from build123d import *

# Parameters (mm, degrees)
CROQUIS1_W              = 50
CROQUIS1_H              = 110
SALIENTE_EXTRUIR1_DEPTH = 4.5
REDONDEO1_R             = 2
CROQUIS2_R              = 3.5
CROQUIS2_R_2            = 2.6
SALIENTE_EXTRUIR2_DEPTH = 5
CROQUIS3_W              = 35
CROQUIS3_H              = 90
SALIENTE_EXTRUIR3_DEPTH = 23
CROQUIS5_W              = 30
CROQUIS5_H              = 21
CORTAR_EXTRUIR2_DEPTH   = 106.61249926
CORTAR_EXTRUIR4_DEPTH   = 10
CORTAR_EXTRUIR5_DEPTH   = 10


with BuildPart() as part:
    # Croquis1 → Saliente-Extruir1 (new body)
    with BuildSketch(Plane.XY):
        Rectangle(CROQUIS1_W, CROQUIS1_H)
    extrude(amount=SALIENTE_EXTRUIR1_DEPTH)

    # Redondeo1
    redondeo1_edges = [part.edges().sort_by_distance(p)[0] for p in [
        (-25, 0, 4.5),
        (0, -55, 4.5),
        (25, 0, 4.5),
        (0, -55, 0),
        (-25, 0, 0),
        (0, 55, 0),
        (25, 0, 0),
        (0, 55, 4.5),
    ]]
    fillet(redondeo1_edges, radius=REDONDEO1_R)

    # Croquis2 → Saliente-Extruir2 (add)
    # profile 1 of 16: a face of its own
    with BuildSketch(Plane.XY.offset(4.5)):
        with Locations(Location((-15, 50, 0), (0, 0, 121.002719134))):
            Circle(CROQUIS2_R)
        with Locations((-15, 50)):
            Circle(CROQUIS2_R_2, mode=Mode.SUBTRACT)
    # profile 2 of 16: a face of its own
    with BuildSketch(Plane.XY.offset(4.5)):
        with Locations((-15, 40)):
            Circle(CROQUIS2_R)
        with Locations((-15, 40)):
            Circle(CROQUIS2_R_2, mode=Mode.SUBTRACT)
    # profile 3 of 16: a face of its own
    with BuildSketch(Plane.XY.offset(4.5)):
        with Locations((-9, 45)):
            Circle(CROQUIS2_R)
        with Locations((-9, 45)):
            Circle(CROQUIS2_R_2, mode=Mode.SUBTRACT)
    # profile 4 of 16: a face of its own
    with BuildSketch(Plane.XY.offset(4.5)):
        with Locations(Location((-21, 45, 0), (0, 0, 235.150095421))):
            Circle(CROQUIS2_R)
        with Locations(Location((-21, 45, 0), (0, 0, 219.715137232))):
            Circle(CROQUIS2_R_2, mode=Mode.SUBTRACT)
    # profile 5 of 16: a face of its own
    with BuildSketch(Plane.XY.offset(4.5)):
        with Locations(Location((21, 45, 0), (0, 0, 180))):
            Circle(CROQUIS2_R)
        with Locations(Location((21, 45, 0), (0, 0, 180))):
            Circle(CROQUIS2_R_2, mode=Mode.SUBTRACT)
    # profile 6 of 16: a face of its own
    with BuildSketch(Plane.XY.offset(4.5)):
        with Locations(Location((15, 40, 0), (0, 0, 180))):
            Circle(CROQUIS2_R)
        with Locations(Location((15, 40, 0), (0, 0, 180))):
            Circle(CROQUIS2_R_2, mode=Mode.SUBTRACT)
    # profile 7 of 16: a face of its own
    with BuildSketch(Plane.XY.offset(4.5)):
        with Locations(Location((9, 45, 0), (0, 0, 180))):
            Circle(CROQUIS2_R)
        with Locations(Location((9, 45, 0), (0, 0, 180))):
            Circle(CROQUIS2_R_2, mode=Mode.SUBTRACT)
    # profile 8 of 16: a face of its own
    with BuildSketch(Plane.XY.offset(4.5)):
        with Locations(Location((15, 50, 0), (0, 0, 180))):
            Circle(CROQUIS2_R)
        with Locations(Location((15, 50, 0), (0, 0, 180))):
            Circle(CROQUIS2_R_2, mode=Mode.SUBTRACT)
    # profile 9 of 16: a face of its own
    with BuildSketch(Plane.XY.offset(4.5)):
        with Locations((15, -40)):
            Circle(CROQUIS2_R)
        with Locations((15, -40)):
            Circle(CROQUIS2_R_2, mode=Mode.SUBTRACT)
    # profile 10 of 16: a face of its own
    with BuildSketch(Plane.XY.offset(4.5)):
        with Locations(Location((21, -45, 0), (0, 0, 55.150095421))):
            Circle(CROQUIS2_R)
        with Locations(Location((21, -45, 0), (0, 0, 39.715137232))):
            Circle(CROQUIS2_R_2, mode=Mode.SUBTRACT)
    # profile 11 of 16: a face of its own
    with BuildSketch(Plane.XY.offset(4.5)):
        with Locations((9, -45)):
            Circle(CROQUIS2_R)
        with Locations((9, -45)):
            Circle(CROQUIS2_R_2, mode=Mode.SUBTRACT)
    # profile 12 of 16: a face of its own
    with BuildSketch(Plane.XY.offset(4.5)):
        with Locations(Location((15, -50, 0), (0, 0, 238.997280866))):
            Circle(CROQUIS2_R)
        with Locations((15, -50)):
            Circle(CROQUIS2_R_2, mode=Mode.SUBTRACT)
    # profile 13 of 16: a face of its own
    with BuildSketch(Plane.XY.offset(4.5)):
        with Locations(Location((-15, -40, 0), (0, 0, 180))):
            Circle(CROQUIS2_R)
        with Locations(Location((-15, -40, 0), (0, 0, 180))):
            Circle(CROQUIS2_R_2, mode=Mode.SUBTRACT)
    # profile 14 of 16: a face of its own
    with BuildSketch(Plane.XY.offset(4.5)):
        with Locations(Location((-9, -45, 0), (0, 0, 180))):
            Circle(CROQUIS2_R)
        with Locations(Location((-9, -45, 0), (0, 0, 180))):
            Circle(CROQUIS2_R_2, mode=Mode.SUBTRACT)
    # profile 15 of 16: a face of its own
    with BuildSketch(Plane.XY.offset(4.5)):
        with Locations(Location((-21, -45, 0), (0, 0, 180))):
            Circle(CROQUIS2_R)
        with Locations(Location((-21, -45, 0), (0, 0, 180))):
            Circle(CROQUIS2_R_2, mode=Mode.SUBTRACT)
    # profile 16 of 16: a face of its own
    with BuildSketch(Plane.XY.offset(4.5)):
        with Locations(Location((-15, -50, 0), (0, 0, 180))):
            Circle(CROQUIS2_R)
        with Locations(Location((-15, -50, 0), (0, 0, 180))):
            Circle(CROQUIS2_R_2, mode=Mode.SUBTRACT)
    extrude(amount=SALIENTE_EXTRUIR2_DEPTH)

    # Croquis3 → Saliente-Extruir3 (add)
    with BuildSketch(Plane(origin=(0, 0, 0), x_dir=(-1, 0, 0), z_dir=(0, 0, -1))):
        Rectangle(CROQUIS3_W, CROQUIS3_H)
    extrude(amount=SALIENTE_EXTRUIR3_DEPTH)

    # Croquis5 → Cortar-Extruir2 (cut, through all)
    with BuildSketch(Plane(origin=(0, 45, 0), x_dir=(1, 0, 0), z_dir=(0, 1, 0))):
        with Locations((0, 11.5)):
            Rectangle(CROQUIS5_W, CROQUIS5_H)
    extrude(amount=-CORTAR_EXTRUIR2_DEPTH, mode=Mode.SUBTRACT)

    # Croquis7 → Cortar-Extruir4 (cut)
    with BuildSketch(Plane.ZY.offset(17.5)):
        with BuildLine():
            add(Edge.make_bspline(
                [(-21.408360481, -7.762503909), (-17.763506305, -12.708708723), (-10.693467631, -23.108472428), (-3.641142742, -7.047797831)],
                knots=[0, 0, 0, 0, 1, 1, 1, 1], degree=3))
            add(Edge.make_bspline(
                [(-21.408360481, -7.762503909), (-21.767705448, -28.605682654), (-0.342880562, -25.676501046), (-3.641142742, -7.047797831)],
                knots=[0, 0, 0, 0, 1, 1, 1, 1], degree=3))
        make_face()
        Polygon((-5.763831244, 18.862685602), (-19.203160033, 12.99310964), (-7.830916468, 3.170101587), align=None)
        Polygon((-14.380375291, 20.063034513), (-16.287856832, 5.033414493), (-3.449369764, 10.442542671), align=None)
        Polygon((-14.380375291, 20.063034513), (-15.047295785, 14.808167615), (-10.611102479, 16.745658244), align=None)
        Polygon((-15.047295785, 14.808167615), (-19.203160033, 12.99310964), (-15.665473408, 9.937360437), align=None)
        Polygon((-12.053495915, 6.817440977), (-15.665473408, 9.937360437), (-16.287856832, 5.033414493), align=None)
        Polygon((-7.074130605, 8.915353688), (-12.053495915, 6.817440977), (-7.830916468, 3.170101587), align=None)
        Polygon((-5.763831244, 18.862685602), (-10.611102479, 16.745658244), (-6.517294779, 13.142655438), align=None)
        Polygon((-6.517294779, 13.142655438), (-7.074130605, 8.915353688), (-3.449369764, 10.442542671), align=None)
    extrude(amount=-CORTAR_EXTRUIR4_DEPTH, mode=Mode.SUBTRACT)

    # Croquis8 → Cortar-Extruir5 (cut)
    with BuildSketch(Plane(origin=(17.5, 0, 0), x_dir=(0, 0, -1), z_dir=(1, 0, 0))):
        with BuildLine():
            add(Edge.make_bspline(
                [(2.569348743, 40.716245485), (9.080503754, 18.53762373), (10.580801765, -9.48585487), (2.377628668, -42.298547258)],
                knots=[0, 0, 0, 0, 1, 1, 1, 1], degree=3))
            add(Edge.make_bspline(
                [(2.377628668, -42.298547258), (5.133604453, -15.937039747), (3.893375388, 16.552759214), (2.569348743, 40.716245485)],
                knots=[0, 0, 0, 0, 1, 1, 1, 1], degree=3))
        make_face()
        with BuildLine():
            add(Edge.make_bspline(
                [(20.430651257, 40.716245485), (13.919496246, 18.53762373), (12.419198235, -9.48585487), (20.622371332, -42.298547258)],
                knots=[0, 0, 0, 0, 1, 1, 1, 1], degree=3))
            add(Edge.make_bspline(
                [(20.622371332, -42.298547258), (17.866395547, -15.937039747), (19.106624612, 16.552759214), (20.430651257, 40.716245485)],
                knots=[0, 0, 0, 0, 1, 1, 1, 1], degree=3))
        make_face()
    extrude(amount=-CORTAR_EXTRUIR5_DEPTH, mode=Mode.SUBTRACT)


solid = part.part
The listing builds one solid part. Answer for the finished solid, in the listing's coordinates (mm). A direction names the side the tool comes from. Coordinates: 2 decimals unless noted, no trailing zeros. Write each loop counter-clockwise with the first axis right and the second up, starting at its lowest first coordinate (ties: lowest second). Pieces come first, ordered by that corner, then holes. Notation, with made-up numbers: M 19.5,75 L 50.5,75 A19 cw 50.5,79 Z; hole C -38,60 d7. An arc over 180 degrees is marked long. Write each question's results on one line, items separated by ' | '.
Item 1: Consider probe 1 along Z at (x, y) = (5.5, 40); probe 2 along Z at (x, y) = (6, 43.5); probe 3 along X at (y, z) = (-32, -8). Determine where each line is inside the solid, lowest interval first. Write a range as [from, to].
Answer below:
probe 1: [-23, -22], [-1, 4.5] | probe 2: [-23, -22], [-1, 9.5] | probe 3: [-17.5, -15], [15, 17.5]
Item 2: Which of the six approach directions +Z, -Z, +X, -X, +Y, -Y give full straight-line access (tool end or side, diameter ignored) to faces 3 (the face through (-16.27, 17.47, -14.71)), 4 (the face through (15, -37, 9.5)), 5 (the face through (-15, 1, -11)), 6 (the face through (21.46, 41.53, 6.96))?
Answer below:
face 3: -X | face 4: +Z, +X, -X, +Y, -Y | face 5: +Y, -Y | face 6: +Z
Item 3: For a pull along Y with two mould halves and no side action, classify faces 1 (the face through (22.19, -47.31, 6.96)), 2 (the face through (24.43, 0.77, 0.6)) as released by +Y, released by -Y, zero draft, split by the parting line, or undercut.
Answer below:
face 1: undercut | face 2: zero draft
Item 4: The part is cut by section D-D on x = -21. Determine the outline of the cut face in (y, z), and give its area (3 significant figures).
Answer below:
outline: M -55,2 A2 ccw -53,0 L 53,0 A2 ccw 55,2 L 55,2.5 A2 ccw 53,4.5 L 48.5,4.5 L 48.5,9.5 L 47.6,9.5 L 47.6,4.5 L 42.4,4.5 L 42.4,9.5 L 41.5,9.5 L 41.5,4.5 L -41.5,4.5 L -41.5,9.5 L -42.4,9.5 L -42.4,4.5 L -47.6,4.5 L -47.6,9.5 L -48.5,9.5 L -48.5,4.5 L -53,4.5 A2 ccw -55,2.5 Z | area: 510 mm2
Item 5: The part is cut by section B-B on y = 50. Determine the outline of the cut face in (x, z).
Answer below:
outline: M -25,2 A2 ccw -23,0 L 23,0 A2 ccw 25,2 L 25,2.5 A2 ccw 23,4.5 L 18.5,4.5 L 18.5,9.5 L 17.6,9.5 L 17.6,4.5 L 12.4,4.5 L 12.4,9.5 L 11.5,9.5 L 11.5,4.5 L -11.5,4.5 L -11.5,9.5 L -12.4,9.5 L -12.4,4.5 L -17.6,4.5 L -17.6,9.5 L -18.5,9.5 L -18.5,4.5 L -23,4.5 A2 ccw -25,2.5 Z
Item 6: Given P1, Ø11.5, axis at x = -6, z = -9, coming from the -Y side (3 decimals); P2, Ø5, axis at x = 0, y = -36, coming from the +Z side; P3, Ø5.5, axis at x = -8.5, y = -44.5, coming from the +Z side; P4, Ø6, axis at y = 19, z = -4, coming from the +X side, each flat-ended and moving along its own axis, determine where each tip first touches the part or whether it passes through.
Answer below:
P1: through | P2: z = 4.5 | P3: z = 9.5 | P4: x = 17.5
Item 7: The part is cut by section C-C on z = 7. State how many separate pieces and enclosed holes the cut face has, and give its area (3 significant figures).
Answer below:
separate pieces: 16 | enclosed holes: 16 | area: 276 mm2
